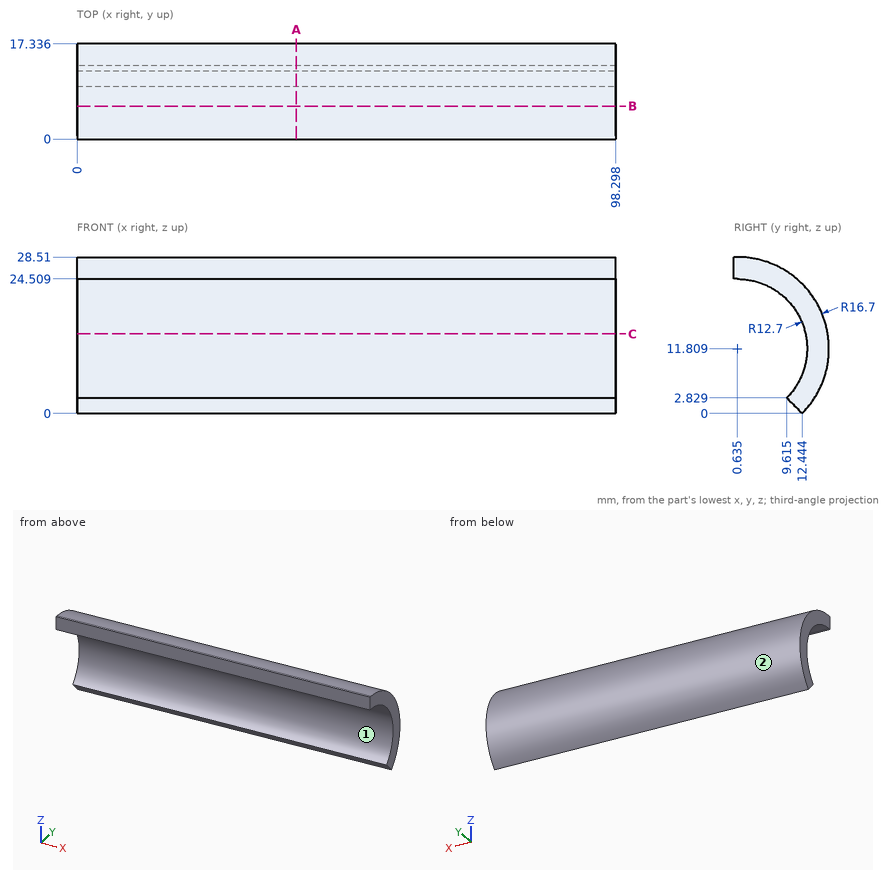
Study the drawing (mm; zero at the part's minimum x, y, z) and answer. Coordinates: 2 decimals unless noted, no trailing zeros. Loops run counter-clockwise (first coordinate to the right, second up) from the corner with the lowest first, then second, coordinate; pieces in that order, holes last. Notation, with made-up numbers: (54, 37.5) -> (85, 37.5) arc R25 cw to (85, 63.5) -> close; hole circle Ø2 at (80.25, 21). An arc over 180 degrees is marked (long way). Answer as CSV lines item,"result".
1) The part is cut by section B-B (y = 6). Give the vertices of the cut face in (x, z) (1 decimal).
A:
outline,"(0, 23.3) -> (98.3, 23.3) -> (98.3, 27.6) -> (0, 27.6) -> close"
2) The part is cut by section A-A (x = 40). Give the vertices of the cut face in (y, z) (1 decimal), and give its area (3 significant figures).
A:
outline,"(0, 24.5) -> (0.6, 24.5) arc R12.7 cw to (9.6, 2.8) -> (12.4, 0) arc R16.7 ccw to (0.6, 28.5) -> (0, 28.5) -> close"
area,"141 mm²"
3) For a pull along Z with two mould halves and no side action, classify the marked faces 1 and 2 as released by +Z, released by -Z, zero draft, split by the parting line, or undercut.
A:
face 1,"undercut"
face 2,"split by the parting line"
4) Straight lines are drawn through the part: probe 1 along Z at (x, y) = (58.5, 10.75) (1 decimal); probe 2 along Y at (x, z) = (8, 11.5); probe 3 along Z at (x, y) = (29, 3.75) (1 decimal). For each, find the intervals that lie inside material, in ascending order.
A:
probe 1,"z = 1.7 to 4.1, 19.5 to 25.1"
probe 2,"y = 13.33 to 17.33"
probe 3,"z = 24.1 to 28.2"
5) Flat-ended cylindrical pins translate along their axes: pin 1 (4 mm diameter, centred on x = 85, z = 15.5, fed in from +Y); pin 2 (6 mm diameter, centred on x = 16.5, y = 8, fed in from +Z); pin 3 (6 mm diameter, centred on x = 15, y = 2, fed in from -Z) (1 decimal). Find the tip coordinate at first contact, or state that the pin passes through.
A:
pin 1,"stops at y = 17.25"
pin 2,"stops at z = 27.93"
pin 3,"stops at z = 23.7"
6) The part is cut by section C-C (z = 14.5). Give the vertices of the cut face in (x, y).
A:
outline,"(0, 13.05) -> (98.3, 13.05) -> (98.3, 17.12) -> (0, 17.12) -> close"
